Design review of the part shown in the three views and the two pictorial views. Dimensions are in mm from the part's minimum x, y and z. A direction names the side the tool comes from. Coordinates: 2 decimals unless noted, no trailing zeros. Order: outer loops, then holes, each group sorted by start corner. A loop starts at its lowest first (then second) coordinate and runs counter-clockwise, first axis right, second up. Notation, with made-up numbers: (-22, -12) -> (7, -12) arc R9 cw to (7, -4) -> close; hole circle Ø11 at (-12, -32). An arc over 180 degrees is marked (long way). Answer as a JSON object with one key per item and string values. Group by question number.
1) Add section B-B, the plane z = 33. Write out the cut boundary in (x, y).
2) Add section A-A, the plane x = 35.5. Write out the cut boundary in (y, z).
3) Machinability: for the marked faces 4 and 5, which of the approach directions +Z, -Z, +X, -X, +Y, -Y give a long, thin tool a straight path to every point of the face, cutting with its end or side? Answer none if there is none.
4) Wall thickness on L1, parallel to Z at x = 45, y = 1.25; L2, parallel to X at y = 7.25, z = 33: over which ranges is each line inside the solid? List them lowest first.
5) Draft analysis for pull direction Z (two halves, no side actions). For the marked faces 1, 2 and 3, state which applies: +Z half, -Z half, draft (parallel to the pull), parting line (faces both ways), or undercut.
6) Add section C-C, the plane y = 2. Write out the cut boundary in (x, z).
7) For pin 1 (2 mm diameter, centred on x = 48.5, z = 27, fed in from +Y); pin 2 (3 mm diameter, centred on y = 7, z = 28, fed in from -X); pin 3 (1.2 mm diameter, centred on x = 27, z = 49, fed in from -Y), all flat-tipped, find the tip position at first contact; note any pin that passes through.
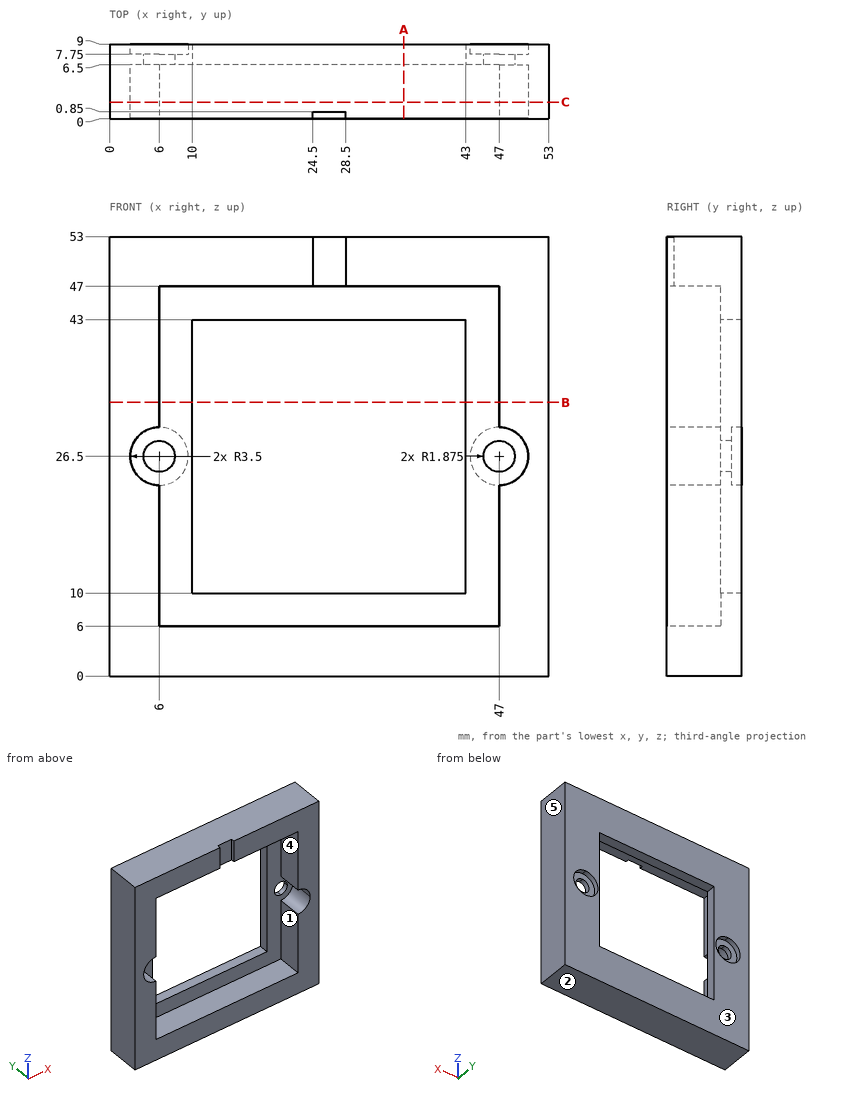
Output values:
{
 "1": {"outline": "(0, 0) -> (6, 0) -> (6, 6.5) -> (10, 6.5) -> (10, 9) -> (0, 9) -> close; (43, 6.5) -> (47, 6.5) -> (47, 0) -> (53, 0) -> (53, 9) -> (43, 9) -> close"},
 "2": {"outline": "(0, 0) -> (9, 0) -> (9, 10) -> (6.5, 10) -> (6.5, 6) -> (0, 6) -> close; (0, 47) -> (6.5, 47) -> (6.5, 43) -> (9, 43) -> (9, 53) -> (0, 53) -> close"},
 "3": {"face 4": "-Y", "face 5": "+Z, -Z, +X, +Y, -Y"},
 "4": {"L1": "z = 0 to 6, 47 to 53", "L2": "x = 0 to 10, 43 to 53"},
 "5": {"face 1": "undercut", "face 2": "-Z half", "face 3": "draft"},
 "6": {"outline": "(0, 0) -> (53, 0) -> (53, 53) -> (0, 53) -> close; hole (6, 6) -> (47, 6) -> (47, 23) arc R3.5 ccw to (47, 30) -> (47, 47) -> (6, 47) -> (6, 30) arc R3.5 ccw to (6, 23) -> close"},
 "7": {"pin 1": "stops at y = 7.75", "pin 2": "stops at x = 0", "pin 3": "stops at y = 0.85"}
}
